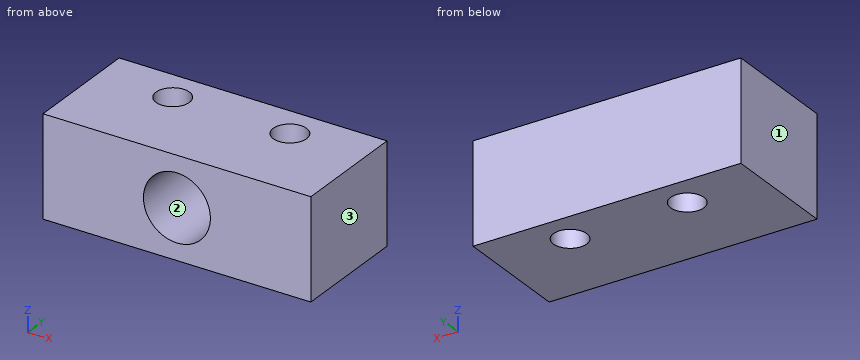
```python
from build123d import *

# Parameters (mm, degrees)
SKETCH_1_W          = 16
SKETCH_1_H          = 10
EXTRUDE_1_DEPTH     = 3
SKETCH_2_R          = 2
CUT_EXTRUDE_1_DEPTH = 5
SKETCH_4_R          = 1
CUT_EXTRUDE_2_DEPTH = 10
SKETCH_5_W          = 20.147345776
SKETCH_5_H          = 7.992609138
CUT_EXTRUDE_3_DEPTH = 3


with BuildPart() as part:
    # 스케치1 → 보스-돌출1 (new, symmetric)
    with BuildSketch(Plane.XY):
        Rectangle(SKETCH_1_W, SKETCH_1_H)
    extrude(amount=EXTRUDE_1_DEPTH, both=True)

    # 스케치2 → 컷-돌출1 (cut)
    with BuildSketch(Plane.XZ.offset(5)):
        with Locations(Location((0, 0, 0), (0, 0, 270))):
            Circle(SKETCH_2_R)
    extrude(amount=-CUT_EXTRUDE_1_DEPTH, mode=Mode.SUBTRACT)

    # 스케치4 → 컷-돌출2 (cut)
    with BuildSketch(Plane.XY.offset(3)):
        with Locations((-3.5, 0)):
            Circle(SKETCH_4_R)
        with Locations((3.5, 0)):
            Circle(SKETCH_4_R)
    extrude(amount=-CUT_EXTRUDE_2_DEPTH, mode=Mode.SUBTRACT)

    # 스케치5 → 컷-돌출3 (cut)
    with BuildSketch(Plane(origin=(0, 5, 0), x_dir=(1, 0, 0), z_dir=(0, 1, 0))):
        Rectangle(SKETCH_5_W, SKETCH_5_H)
    extrude(amount=-CUT_EXTRUDE_3_DEPTH, mode=Mode.SUBTRACT)


solid = part.part
```
Here's how the part is built. I have some questions about the finished solid (model axes, mm). Face numbers are marked on the shaded views. Coordinates: 2 decimals unless noted, no trailing zeros. Loops run counter-clockwise (first coordinate to the right, second up) from the corner with the lowest first, then second, coordinate; pieces in that order, holes last. Notation, with made-up numbers: (5.25, -11.75) - (34.25, -11.75) arc R20 cw to (34.25, 0.25) - close; hole circle Ø7 at (16, 1). An arc over 180 degrees is marked (long way). Return JSON: item names as keys, results as strings. Group by question number.
Item 1: If we section it at A-A on z = 0: Write out the boundary of the cut face in (x, y), and give its area (3 significant figures).
Item 2: Will this pin go through, and if not, where does the flat tip stop? P1, Ø3.5, axis at x = 0, z = 0, coming from the -Y side.
Item 3: I need wall thicknesses on line 1 (X direction, y = -3.7, z = 0); line 2 (X direction, y = -0.25, z = 2.1); line 3 (Y direction, x = -3.5, z = -1.2). Which ranges of each line are inside material? Lowest first, please. Write a range as from..to.
Item 4: If we section it at C-C on y = -0.75: Write out the boundary of the cut face in (x, z), and give its area (3 significant figures).
Item 5: We'd pull the mould along X, two halves only. Please class the marked faces 1, 2 and 3: +X half, -X half, draft (parallel to the pull), parting line (faces both ways), or undercut.
Item 6: If we section it at B-B on x = -3.5: Write out the boundary of the cut face in (y, z).
Item 7: If we section it at D-D on x = 0: Write out the boundary of the cut face in (y, z), and give its area (3 significant figures).
Calculated:
{
 "1": {"outline": "(-8, -5) - (-2, -5) - (-2, 0) - (2, 0) - (2, -5) - (8, -5) - (8, 2) - (-8, 2) - close; hole circle Ø2 at (-3.5, 0); hole circle Ø2 at (3.5, 0)", "area": "85.7 mm^2"},
 "2": {"P1": "stops at y = 0"},
 "3": {"line 1": "x = -8..-2, 2..8", "line 2": "x = -8..-4.47, -2.53..2.53, 4.47..8", "line 3": "y = -5..-1, 1..2"},
 "4": {"outline": "(-8, -3) - (-4.16, -3) - (-4.16, 3) - (-8, 3) - close; (-2.84, -3) - (2.84, -3) - (2.84, 3) - (-2.84, 3) - close; (4.16, -3) - (8, -3) - (8, 3) - (4.16, 3) - close; hole circle Ø4 at (0, 0)", "area": "67.6 mm^2"},
 "5": {"face 1": "-X half", "face 2": "undercut", "face 3": "+X half"},
 "6": {"outline": "(-5, -3) - (-1, -3) - (-1, 3) - (-5, 3) - close; (1, -3) - (2, -3) - (2, 3) - (1, 3) - close"},
 "7": {"outline": "(-5, -3) - (2, -3) - (2, 3) - (-5, 3) - (-5, 2) - (0, 2) - (0, -2) - (-5, -2) - close", "area": "22.0 mm^2"}
}
